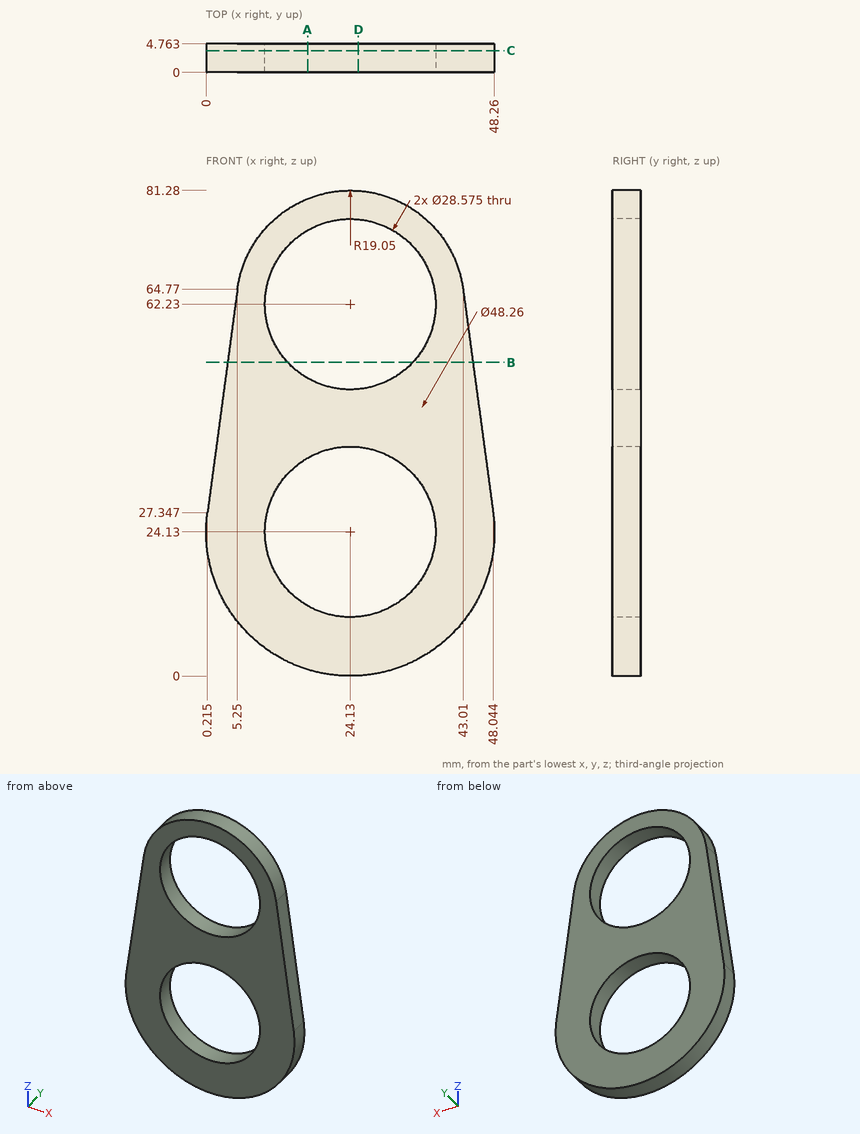
Source: three-view drawing plus pictorial views. Frame: mm from the lowest corner of the part. Give positions to 0.01 mm unless a question says otherwise; leave off trailing zeros. Loops run counter-clockwise (first coordinate to the right, second up) from the corner with the lowest first, then second, coordinate; pieces in that order, holes last.
1) Section query C-C on y = 3.65. Count the separate pieces of the cut face and the enclosed holes in it, and give its area (3 significant figures).
A:
separate pieces: 1
enclosed holes: 2
area: 1,860 mm2
2) Contact query for flat-ended pins moving along their axis: pin 1 (1 mm diameter, centred on y = 1.5, z = 56, fed in from -X); pin 2 (1 mm diameter, centred on y = 1.5, z = 59.5, fed in from -X); pin 3 (2 mm diameter, centred on y = 1.5, z = 63, fed in from +X); pin 4 (17 mm diameter, centred on x = 24.13, z = 62.23, fed in from -Y). Output: stop coordinate, or through.
A:
pin 1: stops at x = 4
pin 2: stops at x = 4.47
pin 3: stops at x = 43.38
pin 4: passes through
3) Section query D-D on x = 25.5. Return the cut outline in (y, z), and give its area (3 significant figures).
A:
outline: (0, 0.04) - (4.76, 0.04) - (4.76, 9.91) - (0, 9.91) - close; (0, 38.35) - (4.76, 38.35) - (4.76, 48.01) - (0, 48.01) - close; (0, 76.45) - (4.76, 76.45) - (4.76, 81.23) - (0, 81.23) - close
area: 116 mm2
4) Section query B-B on z = 52.5. Return the cut outline in (x, y).
A:
outline: (3.6, 0) - (13.67, 0) - (13.67, 4.76) - (3.6, 4.76) - close; (34.59, 0) - (44.66, 0) - (44.66, 4.76) - (34.59, 4.76) - close
5) Section query A-A on x = 17. Return the cut outline in (y, z) (1 decimal).
A:
outline: (0, 1.1) - (4.8, 1.1) - (4.8, 11.7) - (0, 11.7) - close; (0, 36.5) - (4.8, 36.5) - (4.8, 49.8) - (0, 49.8) - close; (0, 74.6) - (4.8, 74.6) - (4.8, 79.9) - (0, 79.9) - close
6) Line query: L1, parallel to Z at x = 22, y = 2.2 (1 decimal); L2, parallel to Z at x = 31, y = 1.35; L3, parallel to X at y = 4.05, z = 21 (1 decimal). Output: solid intervals per line, ascending.
A:
L1: z = 0.1 to 10, 38.3 to 48.1, 76.4 to 81.2
L2: z = 1 to 11.6, 36.66 to 49.7, 74.76 to 80
L3: x = 0.2 to 10.2, 38.1 to 48.1
